Study the drawing (mm; zero at the part's minimum x, y, z) and answer. A direction names the side the tool comes from. Give positions to 0.01 mm unless a question says otherwise; leave off trailing zeros. Write each loop counter-clockwise with the first axis right and the second up, starting at its lowest first coordinate (ties: lowest second). Pieces come first, ordered by that corner, then holes. Notation, with made-up numbers: (-21.75, -14.5) -> (1.25, -14.5) arc R33 ccw to (1.25, 16.5) -> close; hole circle Ø4 at (8, -20.75). An arc over 180 degrees is marked (long way). One line per question, with ' | ' between items.
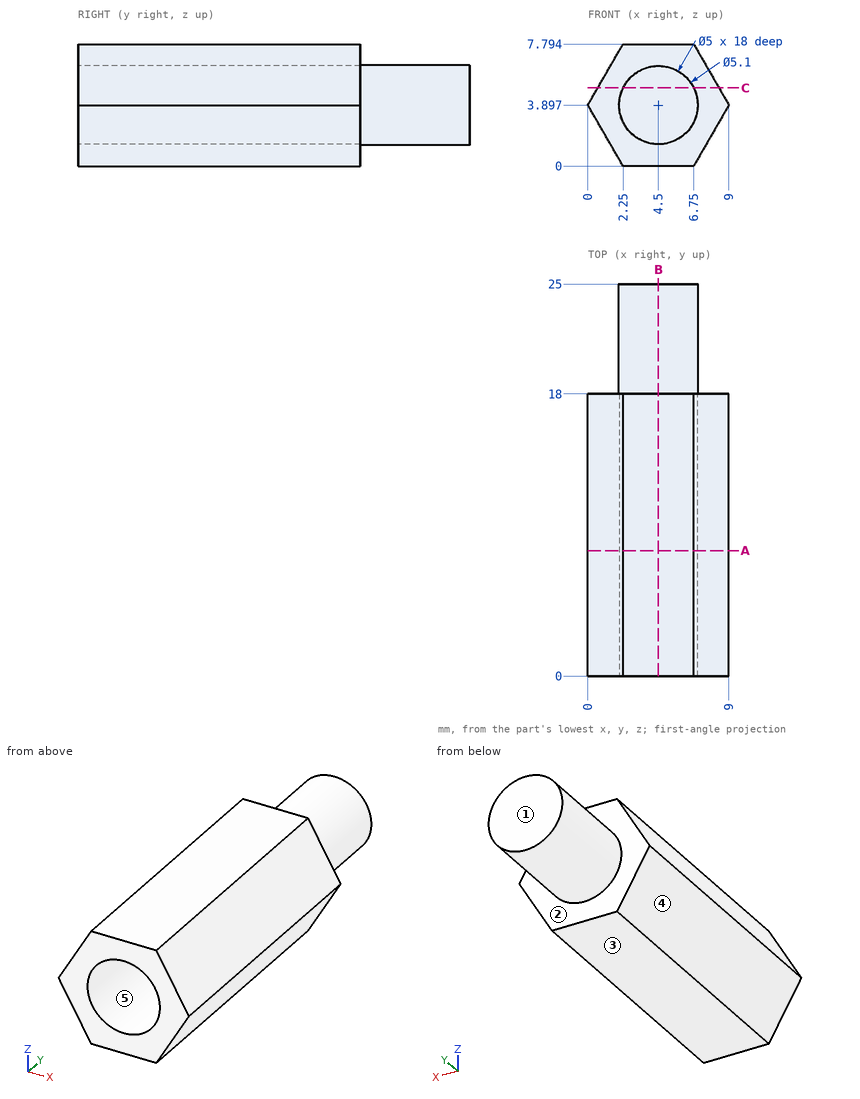
Item 1: Flat-ended cylindrical pins translate along their axes: pin 1 (4 mm diameter, centred on x = 4.5, z = 3.5, fed in from -Y); pin 2 (1 mm diameter, centred on x = 8, y = 16, fed in from -Z); pin 3 (4 mm diameter, centred on y = 8, z = 6.5, fed in from +X). Find the tip coordinate at first contact, or state that the pin passes through.
Answers below:
pin 1: y = 18 | pin 2: z = 1.3 | pin 3: x = 8.65
Item 2: Determine the mould class of the marked faces 3, 4 and 5 for opening direction X: pulls with the +X half, pulls with the -X half, needs draft (parallel to the pull), parting line crosses it, or undercut.
Answers below:
face 3: needs draft | face 4: pulls with the -X half | face 5: undercut
Item 3: A tool of negligible diameter and unlimited length cuts with its end or side. For the marked faces 1 and 2, from which of +Z, -Z, +X, -X, +Y, -Y can it reach the whole face along a straight path? Write none if from no direction.
Answers below:
face 1: +Z, -Z, +X, -X, +Y | face 2: +Y
Item 4: Find section A-A (y = 8). Write down the section's boundary in (x, z), then the cut area to 3 significant figures.
Answers below:
outline: (0, 3.9) -> (2.25, 0) -> (6.75, 0) -> (9, 3.9) -> (6.75, 7.79) -> (2.25, 7.79) -> close; hole circle Ø5 at (4.5, 3.9) | area: 33.0 mm²
Item 5: Find section B-B (x = 4.5). Write down the section's boundary in (y, z).
Answers below:
outline: (0, 0) -> (18, 0) -> (18, 1.35) -> (25, 1.35) -> (25, 6.45) -> (18, 6.45) -> (18, 7.79) -> (0, 7.79) -> (0, 6.4) -> (18, 6.4) -> (18, 1.4) -> (0, 1.4) -> close
Item 6: Find section C-C (z = 5). Write down the section's boundary in (x, y).
Answers below:
outline: (0.64, 0) -> (2.26, 0) -> (2.26, 18) -> (6.74, 18) -> (6.74, 0) -> (8.36, 0) -> (8.36, 18) -> (6.8, 18) -> (6.8, 25) -> (2.2, 25) -> (2.2, 18) -> (0.64, 18) -> close
Item 7: Consider line 1 (Z direction, x = 4.5, y = 12.5); line 2 (Y direction, x = 7.5, z = 1.75); line 3 (Y direction, x = 5.5, z = 5.25). Determine where each line is inside the solid, lowest interval first. Write a range as [from, to].
Answers below:
line 1: [0, 1.4], [6.4, 7.79] | line 2: [0, 18] | line 3: [18, 25]
